Input: part model. Units: mm. Frame: model coordinates. Coordinates: 2 decimals unless noted, no trailing zeros. Loops run counter-clockwise (first coordinate to the right, second up) from the corner with the lowest first, then second, coordinate; pieces in that order, holes last. Notation, with made-up numbers: M 11,85.25 L 27,85.25 A7 ccw 27,92.25 Z; hole C 43.25,-7 d7. An arc over 180 degrees is marked long. Use a Markdown table: item, result. Add a question column.
1. Section C-C on z = 7. Output: boundary loops of the cut face in (x, y) (3 decimals), then the cut area to 4 significant figures.
2. Section B-B on x = 0. Output: boundary loops of the cut face in (y, z) (3 decimals), then the cut area to 3 significant figures.
3. Section A-A on z = 0. Output: boundary loops of the cut face in (x, y) (3 decimals).
4. Pin query (flat end, axial travel): pin 1 (2 mm diameter, centred on x = 0, z = -7, fed in from +Y); pin 2 (0.5 mm diameter, centred on y = 3.5, z = 16.5, fed in from +X); pin 3 (6 mm diameter, centred on x = 7, z = -6, fed in from +Y); pin 4 (0.6 mm diameter, centred on x = -1, y = 5.5, fed in from -Z). Return the tip coordinate at first contact, or that it passes through.
5. Line query: L1, parallel to X at y = 3.25, z = 0 (3 decimals); L2, parallel to Z at x = 0.75, y = 2.5; L3, parallel to X at y = 2.95, z = 7 (3 decimals). Output: solid intervals per line, ascending. Write a range as [from, to].
6. Section D-D on y = 4.2. State how many separate pieces and enclosed holes the cut face has, then the cut area to 3 significant figures.
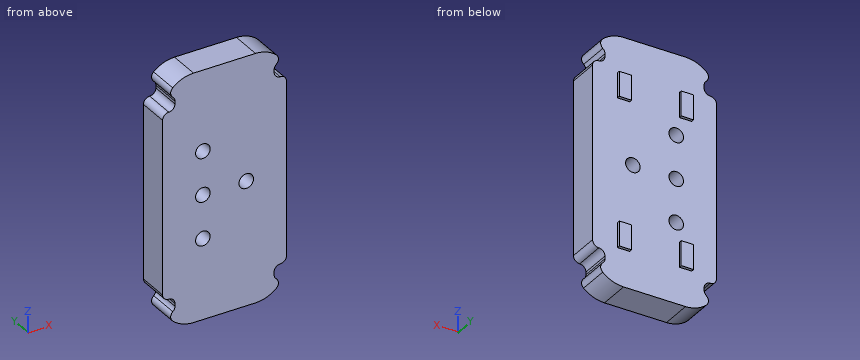
```python
from build123d import *

# Parameters (mm, degrees)
SKETCH1_W            = 20
SKETCH1_H            = 40
SKETCH1_R            = 1.175
BOSS_EXTRUDE1_DEPTH  = 5
FILLET1_R            = 5
SKETCH2_W            = 2
SKETCH2_H            = 4
BOSS_EXTRUDE2_DEPTH  = 0.5
LPATTERN1_COUNT      = 2
LPATTERN1_PITCH      = 10
LPATTERN1_COUNT_DIR2 = 2
LPATTERN1_PITCH_DIR2 = 24
CUT_EXTRUDE1_DEPTH   = 25.748737342
FILLET2_R            = 1


with BuildPart() as part:
    # Sketch1 → Boss-Extrude1 (new body)
    with BuildSketch(Plane(origin=(0, 0, 0), x_dir=(1, 0, 0), z_dir=(0, 1, 0))):
        with Locations((3.5, 0)):
            Rectangle(SKETCH1_W, SKETCH1_H)
        with Locations(Location((0, 0, 0), (0, 0, 270))):
            Circle(SKETCH1_R, mode=Mode.SUBTRACT)
        with Locations(Location((0, 7, 0), (0, 0, 270))):
            Circle(SKETCH1_R, mode=Mode.SUBTRACT)
        with Locations(Location((7, 0, 0), (0, 0, 270))):
            Circle(SKETCH1_R, mode=Mode.SUBTRACT)
        with Locations(Location((0, -7, 0), (0, 0, 270))):
            Circle(SKETCH1_R, mode=Mode.SUBTRACT)
    extrude(amount=BOSS_EXTRUDE1_DEPTH)

    # Fillet1
    fillet1_edges = [part.edges().sort_by_distance(p)[0] for p in [
        (-6.5, 2.5, -20),
        (13.5, 2.5, -20),
        (13.5, 2.5, 20),
        (-6.5, 2.5, 20),
    ]]
    fillet(fillet1_edges, radius=FILLET1_R)

    # Sketch2 → Boss-Extrude2 (add)
    with BuildSketch(Plane(origin=(0, 5, 0), x_dir=(1, 0, 0), z_dir=(0, 1, 0))):
        with Locations((-1.5, 12)):
            Rectangle(SKETCH2_W, SKETCH2_H)
    boss_extrude2 = extrude(amount=BOSS_EXTRUDE2_DEPTH)

    # LPattern1: Boss-Extrude2 2 × 2
    with Locations(*[(i * LPATTERN1_PITCH, 0, j * LPATTERN1_PITCH_DIR2) for i in range(LPATTERN1_COUNT) for j in range(LPATTERN1_COUNT_DIR2) if (i, j) != (0, 0)]):
        add(boss_extrude2)

    # Sketch4 → Cut-Extrude1 (cut, through all)
    with BuildSketch(Plane.XZ):
        with BuildLine():
            Line((-7.54955844, 17.440393275), (-5.5, 17.440393275))
            ThreePointArc((-5.5, 17.440393275), (-4.792893219, 17.147500056), (-4.5, 16.440393275))
            Line((-4.5, 16.440393275), (-4.5, 16))
            ThreePointArc((-4.5, 16), (-4.792893219, 15.292893219), (-5.5, 15))
            Line((-5.5, 15), (-7.54955844, 15))
            Line((-7.54955844, 15), (-7.54955844, 17.440393275))
        make_face()
        with BuildLine():
            Line((14.54955844, 17.440393275), (14.54955844, 15))
            Line((14.54955844, 15), (12.5, 15))
            ThreePointArc((12.5, 15), (11.792893219, 15.292893219), (11.5, 16))
            Line((11.5, 16), (11.5, 16.440393275))
            ThreePointArc((11.5, 16.440393275), (11.792893219, 17.147500056), (12.5, 17.440393275))
            Line((12.5, 17.440393275), (14.54955844, 17.440393275))
        make_face()
        with BuildLine():
            Line((14.54955844, -17.440393275), (12.5, -17.440393275))
            ThreePointArc((12.5, -17.440393275), (11.792893219, -17.147500056), (11.5, -16.440393275))
            Line((11.5, -16.440393275), (11.5, -16))
            ThreePointArc((11.5, -16), (11.792893219, -15.292893219), (12.5, -15))
            Line((12.5, -15), (14.54955844, -15))
            Line((14.54955844, -15), (14.54955844, -17.440393275))
        make_face()
        with BuildLine():
            Line((-4.5, -16.440393275), (-4.5, -16))
            ThreePointArc((-4.5, -16), (-4.792893219, -15.292893219), (-5.5, -15))
            Line((-5.5, -15), (-7.54955844, -15))
            Line((-7.54955844, -15), (-7.54955844, -17.440393275))
            Line((-7.54955844, -17.440393275), (-5.5, -17.440393275))
            ThreePointArc((-5.5, -17.440393275), (-4.792893219, -17.147500056), (-4.5, -16.440393275))
        make_face()
    extrude(amount=-CUT_EXTRUDE1_DEPTH, mode=Mode.SUBTRACT)

    # Fillet2
    fillet2_edges = [part.edges().sort_by_distance(p)[0] for p in [
        (12.863998243, 2.5, -17.440393275),
        (13.5, 2.5, -15),
        (-5.863998243, 2.5, -17.440393275),
        (-6.5, 2.5, -15),
        (13.5, 2.5, 15),
        (12.863998243, 2.5, 17.440393275),
        (-6.5, 2.5, 15),
        (-5.863998243, 2.5, 17.440393275),
    ]]
    fillet(fillet2_edges, radius=FILLET2_R - 0.0001)  # a hair under: the kernel refuses the full size


solid = part.part
```
Answers below:
| question | item | result |
|---|---|---|
| 1 | outline | M -6.5,0 L -1.175,0 L -1.175,5 L -6.5,5 Z; M 1.175,0 L 13.5,0 L 13.5,5 L 1.175,5 Z |
| 1 | area | 88.25 mm² |
| 2 | outline | M 0,-20 L 5,-20 L 5,-8.175 L 0,-8.175 Z; M 0,-5.825 L 5,-5.825 L 5,-1.175 L 0,-1.175 Z; M 0,1.175 L 5,1.175 L 5,5.825 L 0,5.825 Z; M 0,8.175 L 5,8.175 L 5,20 L 0,20 Z |
| 2 | area | 165 mm² |
| 3 | outline | M -6.5,0 L -1.175,0 L -1.175,5 L -6.5,5 Z; M 1.175,0 L 5.825,0 L 5.825,5 L 1.175,5 Z; M 8.175,0 L 13.5,0 L 13.5,5 L 8.175,5 Z |
| 4 | pin 1 | passes through |
| 4 | pin 2 | stops at x = 11.55 |
| 4 | pin 3 | stops at y = 5 |
| 4 | pin 4 | stops at z = -14 |
| 5 | L1 | x = [-6.5, -1.175], [1.175, 5.825], [8.175, 13.5] |
| 5 | L2 | z = [-20, -7.9], [-6.1, -0.9], [0.9, 6.1], [7.9, 20] |
| 5 | L3 | x = [-6.5, -1.175], [1.175, 13.5] |
| 6 | separate pieces | 1 |
| 6 | enclosed holes | 4 |
| 6 | area | 743 mm² |
